Model file for the job. Use its own axes, mm. Face numbers are marked on the shaded views. Give positions to 0.01 mm unless a question says otherwise; leave off trailing zeros. Order: outer loops, then holes, each group sorted by start corner. A loop starts at its lowest first (then second) coordinate and runs counter-clockwise, first axis right, second up. Notation, with made-up numbers: (-12, -16.75) - (39, -16.75) arc R9 cw to (39, -1.75) - close; hole circle Ø9 at (64, 72). An arc over 180 degrees is marked (long way). Return JSON: item names as keys, results as strings. Group by question number.
from build123d import *

# Parameters (mm, degrees)
F1_DEPTH      = 250
F2_W          = 272.5
F2_H          = 2
F3_DEPTH      = 37
F5_DEPTH      = 37.001
F6_R          = 2.4
F7_DEPTH      = 25
F7_DEPTH_BACK = 25


with BuildPart() as f1:
    # F0 (on Top) → F1 (new body)
    with BuildSketch(Plane.XY):
        with BuildLine():
            Line((18.5, -290), (18.5, 0))
            ThreePointArc((18.5, 0), (0, 18.5), (-18.5, 0))
            Line((-18.5, 0), (-18.5, -290))
            Line((-18.5, -290), (-17.5, -290))
            Line((-17.5, -290), (-17.5, 0))
            ThreePointArc((-17.5, 0), (-12.3743686708, 12.3743686708), (0, 17.5))
            ThreePointArc((0, 17.5), (12.3743686708, 12.3743686708), (17.5, 0))
            Line((17.5, 0), (17.5, -290))
            Line((17.5, -290), (18.5, -290))
        make_face()
    extrude(amount=F1_DEPTH)

    # F2 (on face) → F3 (join)
    with BuildSketch(Plane(origin=(-18.5, 0, 0), x_dir=(0, -1, 0), z_dir=(-1, 0, 0))):
        with Locations((153.75, 1)):
            Rectangle(F2_W, F2_H)
    extrude(amount=-F3_DEPTH)

    # F4 (on face) → F5 (cut, through all)
    with BuildSketch(Plane(origin=(-18.5, 0, 0), x_dir=(0, -1, 0), z_dir=(-1, 0, 0))):
        with BuildLine():
            ThreePointArc((240, 60), (200, 100), (160, 60))
            Line((160, 60), (240, 60))
        make_face()
        with BuildLine():
            Line((240, 60), (160, 60))
            ThreePointArc((160, 60), (200, 20), (240, 60))
        make_face()
        with BuildLine():
            ThreePointArc((67, 175), (70, 172), (73, 175))
            Line((73, 175), (67, 175))
        make_face()
        with BuildLine():
            Line((67, 175), (73, 175))
            ThreePointArc((73, 175), (70, 178), (67, 175))
        make_face()
    extrude(amount=-F5_DEPTH, mode=Mode.SUBTRACT)

    # F6 (on Right) → F7 (cut, two sides)
    with BuildSketch(Plane.YZ) as f7_sk:
        with Locations((-10, 20)):
            Circle(F6_R)
        with Locations((10, 20)):
            Circle(F6_R)
        with Locations((-10, 125)):
            Circle(F6_R)
        with BuildLine():
            ThreePointArc((12.4, 125), (10, 127.4), (7.6, 125))
            ThreePointArc((7.6, 125), (10, 122.6), (12.4, 125))
        make_face()
        with Locations((10, 230)):
            Circle(F6_R)
        with Locations((-10, 230)):
            Circle(F6_R)
    extrude(amount=-F7_DEPTH, mode=Mode.SUBTRACT)
    extrude(f7_sk.sketch, amount=F7_DEPTH_BACK, mode=Mode.SUBTRACT)


solid = f1.part
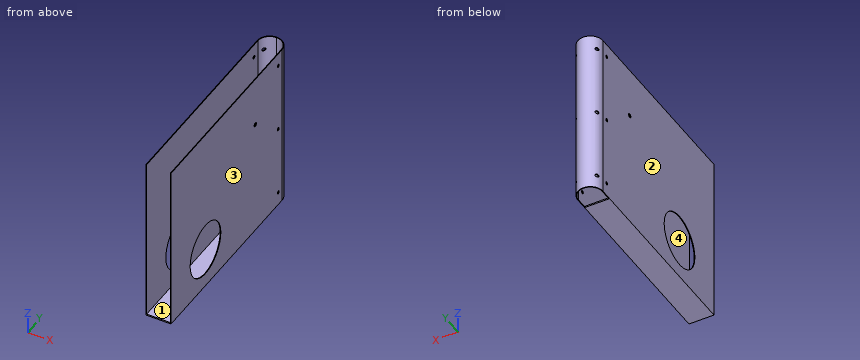
(1) Slice it at A-A (z = 60). Give the cut face in (x, y).
(2) Slice it at C-C (x = -8). Give the cut face in (y, z).
(3) Drill centre lines: L1, parallel to X at y = -271, z = 171; L2, parallel to Z at x = 17.85, y = -10; L3, parallel to Z at x = -18.15, y = -200. Where is each one in solid material? Low to high.
(4) Drop flat-ended pins along their axis: pin 1 Ø1.5 at (x, z) = (7, 148) entering from +Y; pin 2 Ø3 at (x, y) = (-10, -166.5) entering from +Z; pin 3 Ø3 at (x, z) = (10, 147) entering from +Y; pin 4 Ø7.5 at (y, z) = (-10, 125) entering from -X. Give the stop position or say it passes through.
(5) Pull direction X, two halves, no side cores. Call the marked faces 1, 2, 3 and 4: released by +X, released by -X, zero draft, split by the parting line, or undercut.
(6) Slice it at B-B (y = -200). Give the cut face in (x, z).
(7) Slice it at D-D (y = -59.5). Give the cut face in (x, z).
Result set:
{
 "1": {"outline": "(-18.5, -290) - (-17.5, -290) - (-17.5, -240) - (-18.5, -240) - close; (-18.5, -160) - (-17.5, -160) - (-17.5, 0) arc R17.5 cw to (17.5, 0) - (17.5, -160) - (18.5, -160) - (18.5, 0) arc R18.5 ccw to (-18.5, 0) - close; (17.5, -290) - (18.5, -290) - (18.5, -240) - (17.5, -240) - close"},
 "2": {"outline": "(-290, 0) - (-17.5, 0) - (-17.5, 2) - (-290, 2) - close; (15.56, 0) - (16.68, 0) - (16.68, 250) - (15.56, 250) - close"},
 "3": {"L1": "x = -18.5 to -17.5, 17.5 to 18.5", "L2": "z = 0 to 17.6, 22.4 to 122.6, 127.4 to 227.6, 232.4 to 250", "L3": "z = 0 to 20, 100 to 250"},
 "4": {"pin 1": "stops at y = 17.41", "pin 2": "stops at z = 2", "pin 3": "stops at y = 16.43", "pin 4": "stops at x = -18.5"},
 "5": {"face 1": "undercut", "face 2": "released by -X", "face 3": "released by +X", "face 4": "undercut"},
 "6": {"outline": "(-18.5, 0) - (18.5, 0) - (18.5, 20) - (17.5, 20) - (17.5, 2) - (-17.5, 2) - (-17.5, 20) - (-18.5, 20) - close; (-18.5, 100) - (-17.5, 100) - (-17.5, 250) - (-18.5, 250) - close; (17.5, 100) - (18.5, 100) - (18.5, 250) - (17.5, 250) - close"},
 "7": {"outline": "(-18.5, 0) - (18.5, 0) - (18.5, 250) - (17.5, 250) - (17.5, 2) - (-17.5, 2) - (-17.5, 250) - (-18.5, 250) - close"}
}
